Autodesk Inventor part; units mm, degrees
ref_plane "РабПлоскость1" through (-34.9448, 28.465, -130.3508) normal (0, 0, 1) x (1, 0, 0)
ref_plane "YZ Plane" through (0, 0, 0) normal (1, 0, 0) x (0, 1, 0)
ref_plane "XZ Plane" through (0, 0, 0) normal (0, 1, 0) x (-1, 0, 0)
ref_plane "РабПлоскость1" through (-34.9448, 28.465, -130.3508) normal (0, 0, 1) x (1, 0, 0)
sketch "Эскиз1" plane through (-34.9448, 28.465, -130.3508) normal (0, 0, 1) x (1, 0, 0)
  line L0 (0, 3.6904) -> (-12.8571, 3.6904) construction
  line L1 (0, 3.6904) -> (0, 9.6905)
  line L2 (-12.8571, 9.6905) -> (0, 9.6905)
  line L3 (-12.8571, 3.6904) -> (-12.8571, 9.6905)
  line L4 (25.7143, 3.6904) -> (12.8571, 3.6904) construction
  line L5 (25.7143, 3.6904) -> (25.7143, 9.6905)
  line L6 (12.8571, 9.6905) -> (25.7143, 9.6905)
  line L7 (12.8571, 3.6904) -> (12.8571, 9.6905)
  line L8 (51.4286, 3.6904) -> (38.5714, 3.6904) construction
  line L9 (51.4286, 3.6904) -> (51.4286, 9.6905)
  line L10 (38.5714, 9.6905) -> (51.4286, 9.6905)
  line L11 (38.5714, 3.6904) -> (38.5714, 9.6905)
  line L12 (77.1429, 3.6904) -> (64.2857, 3.6904) construction
  line L13 (77.1429, 3.6904) -> (77.1429, 9.6905)
  line L14 (64.2857, 9.6905) -> (77.1429, 9.6905)
  line L15 (64.2857, 3.6904) -> (64.2857, 9.6905)
  line L16 (0, 3.6904) -> (12.8571, 3.6904)
  line L17 (25.7143, 3.6904) -> (38.5714, 3.6904)
  line L18 (51.4286, 3.6904) -> (64.2857, 3.6904)
  line L19 (-12.8571, 3.6904) -> (-12.8571, -50.3096)
  line L20 (-9.8571, -53.3096) -> (-4.7353, -53.3096)
  line L21 (77.1429, 3.6904) -> (77.1429, -50.3096)
  line L22 (74.1429, -53.3096) -> (69.021, -53.3096)
  line L23 (-1.8571, -53.3096) -> (66.1429, -53.3096) construction
  arc A0 (-1.7452, -56.0663) -> (66.0309, -56.0663) centre (32.1429, -53.3096) ccw
  arc A1 (-1.7452, -56.0663) -> (-4.7353, -53.3096) centre (-4.7353, -56.3096) ccw
  arc A2 (69.021, -53.3096) -> (66.0309, -56.0663) centre (69.021, -56.3096) ccw
  arc A3 (74.1429, -53.3096) -> (77.1429, -50.3096) centre (74.1429, -50.3096) ccw
  arc A4 (-12.8571, -50.3096) -> (-9.8571, -53.3096) centre (-9.8571, -50.3096) ccw
  circle A5 centre (32.1429, -53.3095) radius 2.375
  point P0 (34.9448, -28.465)
  point P1 (77.1429, -53.3096)
  dimension "d0" = 57
  dimension "d1" = 34
  dimension "d2" = 3
  dimension "d3" = 6
  dimension "d14" = 4.75
ref_plane "РабПлоскость2" through (-162.802, 331.465, 111.3492) normal (0, 0, 1) x (1, 0, 0)
extrude "Выдавливание1" add sketch "Эскиз1" along normal blind 6
sketch "Эскиз6" plane through (-34.9448, 28.465, -130.3508) normal (0, 0, -1) x (-1, 0, 0)
  line L0 (-30.9731, -35.6894) -> (-30.9731, -26.6894)
  line L1 (-30.9731, -26.6894) -> (-26.9731, -26.6894)
  line L2 (-26.9731, -35.6894) -> (-30.9731, -35.6894)
  line L3 (-26.9731, -26.6894) -> (-26.9731, -35.6894)
  line L4 (-26.9731, 0.3106) -> (-26.9731, -8.6894)
  line L5 (-26.9731, -8.6894) -> (-30.9731, -8.6894)
  line L6 (-30.9731, 0.3106) -> (-26.9731, 0.3106)
  line L7 (-30.9731, -8.6894) -> (-30.9731, 0.3106)
extrude "Выдавливание5" cut sketch "Эскиз6" against normal blind 10
sketch "Эскиз2" plane through (-34.9448, 28.465, -130.3508) normal (0, 0, -1) x (-1, 0, 0)
  line L0 (-4.9286, 3.6904) -> (-4.9286, -2.6596)
  line L1 (-4.9286, -2.6596) -> (-3.6786, -2.6596)
  line L2 (-3.6786, -2.6596) -> (-3.6786, -4.9596)
  line L3 (-3.6786, -4.9596) -> (-4.9286, -4.9596)
  line L4 (-4.9286, -4.9596) -> (-4.9286, -11.3096)
  line L5 (-4.9286, -11.3096) -> (-7.9286, -11.3096)
  line L6 (-7.9286, -11.3096) -> (-7.9286, -4.9596)
  line L7 (-7.9286, -4.9596) -> (-9.1786, -4.9596)
  line L8 (-9.1786, -4.9596) -> (-9.1786, -2.6596)
  line L9 (-9.1786, -2.6596) -> (-7.9286, -2.6596)
  line L10 (-7.9286, -2.6596) -> (-7.9286, 3.6904)
  line L11 (-56.3571, 3.6904) -> (-59.3571, 3.6904)
  line L12 (-56.3571, 3.6904) -> (-56.3571, -2.6596)
  line L13 (-56.3571, -2.6596) -> (-55.1071, -2.6596)
  line L14 (-55.1071, -2.6596) -> (-55.1071, -4.9596)
  line L15 (-55.1071, -4.9596) -> (-56.3571, -4.9596)
  line L16 (-56.3571, -4.9596) -> (-56.3571, -11.3096)
  line L17 (-56.3571, -11.3096) -> (-59.3571, -11.3096)
  line L18 (-59.3571, -11.3096) -> (-59.3571, -4.9596)
  line L19 (-59.3571, -4.9596) -> (-60.6071, -4.9596)
  line L20 (-60.6071, -4.9596) -> (-60.6071, -2.6596)
  line L21 (-60.6071, -2.6596) -> (-59.3571, -2.6596)
  line L22 (-59.3571, -2.6596) -> (-59.3571, 3.6904)
  line L23 (-56.3571, 3.6904) -> (-59.3571, 3.6904)
  line L24 (-4.9286, 3.6904) -> (-7.9286, 3.6904)
  line L25 (-25.7143, 3.6904) -> (-25.7143, 9.6905)
  line L26 (-38.5714, 3.6904) -> (-25.7143, 3.6904)
  line L27 (-38.5714, 9.6905) -> (-38.5714, 3.6904)
  line L28 (-51.4286, 3.6904) -> (-51.4286, 9.6905)
  line L29 (-64.2857, 3.6904) -> (-51.4286, 3.6904)
  line L30 (-64.2857, 9.6905) -> (-64.2857, 3.6904)
  line L31 (-77.1429, -50.3096) -> (-77.1429, 9.6905)
  arc A0 (-77.1429, -50.3096) -> (-74.1429, -53.3096) centre (-74.1429, -50.3096) ccw
  line L32 (-69.021, -53.3096) -> (-74.1429, -53.3096)
  arc A1 (-66.0309, -56.0663) -> (-69.021, -53.3096) centre (-69.021, -56.3096) ccw
  arc A2 (-66.0309, -56.0663) -> (1.7452, -56.0663) centre (-32.1429, -53.3096) ccw
  arc A3 (4.7353, -53.3096) -> (1.7452, -56.0663) centre (4.7353, -56.3096) ccw
  line L33 (9.8571, -53.3096) -> (4.7353, -53.3096)
  arc A4 (9.8571, -53.3096) -> (12.8571, -50.3096) centre (9.8571, -50.3096) ccw
  line L34 (12.8571, 9.6905) -> (12.8571, -50.3096)
  line L35 (0, 3.6904) -> (0, 9.6905)
  line L36 (-12.8571, 3.6904) -> (0, 3.6904)
  line L37 (-12.8571, 9.6905) -> (-12.8571, 3.6904)
  circle A5 centre (-32.1429, -53.3095) radius 2.375
  line L38 (-25.7143, 9.6905) -> (-12.8571, 9.6905)
  line L39 (-51.4286, 9.6905) -> (-38.5714, 9.6905)
  line L40 (-77.1429, 9.6905) -> (-64.2857, 9.6905)
  line L41 (0, 9.6905) -> (12.8571, 9.6905)
  point P0 (-6.4286, 0)
sketch "Эскиз4" plane through (29.3409, 38.1554, -130.3508) normal (0, 1, 0) x (1, 0, 0)
  line L0 (-77.1429, 0) -> (-77.1429, -6)
  line L1 (12.8571, 0) -> (-77.1429, 0)
  line L2 (-77.1429, 0) -> (-77.1429, -6)
  line L3 (-77.1429, -6) -> (12.8571, -6)
  line L4 (12.8571, -6) -> (12.8571, 0)
  point P0 (-29.3409, -130.3508)
sketch "Эскиз5" plane through (-34.9448, 28.465, -130.3508) normal (0, 0, -1) x (-1, 0, 0)
  line L0 (-236.4804, 8.6905) -> (-77.1429, 8.6905) construction
  line L1 (-77.1429, 8.6905) -> (-64.2857, 8.6905) construction
  line L2 (-64.2857, 8.6905) -> (-51.4286, 8.6905) construction
  line L3 (-51.4286, 8.6905) -> (-38.5714, 8.6905) construction
  line L4 (-38.5714, 8.6905) -> (-25.7143, 8.6905) construction
  line L5 (-25.7143, 8.6905) -> (-12.8571, 8.6905) construction
  line L6 (-12.8571, 8.6905) -> (0, 8.6905) construction
  line L7 (0, 8.6905) -> (12.8571, 8.6905) construction
  line L8 (12.8571, 8.6905) -> (44.8254, 8.6905) construction
  line L9 (44.8254, 8.6905) -> (44.8254, 3.6905) construction
  line L10 (44.8254, 3.6905) -> (12.8571, 3.6905) construction
  line L11 (12.8571, 3.6905) -> (12.8571, 8.6905) construction
  line L12 (-236.4804, 3.6905) -> (-236.4804, 8.6905) construction
  line L13 (-77.1429, 3.6905) -> (-236.4804, 3.6905) construction
  line L14 (-64.2857, 3.6905) -> (-77.1429, 3.6905) construction
  line L15 (-51.4286, 3.6905) -> (-64.2857, 3.6905) construction
  line L16 (-38.5714, 3.6905) -> (-51.4286, 3.6905) construction
  line L17 (-25.7143, 3.6905) -> (-38.5714, 3.6905) construction
  line L18 (-12.8571, 3.6905) -> (-25.7143, 3.6905) construction
  line L19 (0, 3.6905) -> (-12.8571, 3.6905) construction
  line L20 (12.8571, 3.6905) -> (0, 3.6905) construction
  line L21 (-77.1429, 8.6905) -> (-77.1429, 3.6905) construction
  line L22 (-64.2857, 3.6905) -> (-64.2857, 8.6905) construction
  line L23 (-51.4286, 8.6905) -> (-51.4286, 3.6905) construction
  line L24 (-38.5714, 3.6905) -> (-38.5714, 8.6905) construction
  line L25 (-25.7143, 8.6905) -> (-25.7143, 3.6905) construction
  line L26 (-12.8571, 3.6905) -> (-12.8571, 8.6905) construction
  line L27 (0, 8.6905) -> (0, 3.6905) construction
  line L28 (-242.4804, 3.6905) -> (-352.8338, 3.6905) construction
  line L29 (-352.8338, 3.6905) -> (-352.8338, 8.6905) construction
  line L30 (-352.8338, 8.6905) -> (-242.4804, 8.6905) construction
  line L31 (-242.4804, 8.6905) -> (-242.4804, 3.6905) construction
  line L32 (-34.1429, 3.6915) -> (-30.1429, 3.6915) construction
  line L33 (-30.1429, -50.9345) -> (-34.1429, -50.9345) construction
  line L34 (-34.1429, 3.6915) -> (-30.1429, -50.9345) construction
  line L35 (-30.1429, 3.6915) -> (-34.1429, -50.9345) construction
  circle A0 centre (-32.1429, -53.3095) radius 2.375 construction
  line L36 (-34.1429, -5.6215) -> (-30.1429, -5.6215)
  line L37 (-30.1429, -41.6215) -> (-34.1429, -41.6215)
  line L38 (-34.1429, -5.6215) -> (-30.1429, -41.6215) construction
  line L39 (-30.1429, -5.6215) -> (-34.1429, -41.6215) construction
  line L40 (-34.1429, -14.6215) -> (-30.1429, -14.6215)
  line L41 (-30.1429, -32.6215) -> (-34.1429, -32.6215)
  line L42 (-34.1429, -14.6215) -> (-30.1429, -32.6215) construction
  line L43 (-30.1429, -14.6215) -> (-34.1429, -32.6215) construction
  line L44 (-34.1429, -41.6215) -> (-34.1429, -32.6215)
  line L45 (-34.1429, -14.6215) -> (-34.1429, -5.6215)
  line L46 (-30.1429, -5.6215) -> (-30.1429, -14.6215)
  line L47 (-30.1429, -32.6215) -> (-30.1429, -41.6215)
  line L48 (-30.1429, -32.6215) -> (-30.1429, -41.6215) construction
  line L49 (-34.1429, -50.9345) -> (-34.1429, -32.6215) construction
  line L50 (-34.1429, -14.6215) -> (-34.1429, 3.6915) construction
  line L51 (-30.1429, 3.6915) -> (-30.1429, 3.6905) construction
  line L52 (-30.1429, -5.6215) -> (-30.1429, -14.6215) construction
  point P0 (-34.9448, -28.465)
  point P1 (-32.1429, -23.6215)
  point P2 (-32.1429, -50.9345)
  dimension "d20" = 4
  dimension "d21" = 54.626
equation "\"d4\" = d3"
properties part number "wheel1"
Work out the finished part from the listing and answer in its coordinate system (mm). A direction names the side the tool comes from. Round coordinates to 2 decimals unless told otherwise and drop trailing zeros. Write each loop counter-clockwise with the first axis right and the second up, starting at its lowest first coordinate (ties: lowest second). Pieces come first, ordered by that corner, then holes.
1) A cutting plane is placed at D-D (y = -42). Give the vertices of the cut face in (x, z), plus the area to 3 significant figures.
2) A tool of negligible diameter and unlimited length cuts with its end or side. For faces 1 (the flat face through (-29, 32.155, -127)), 2 (the flat face through (37, -24.845, -127)), 3 (the flat face through (-42, -24.845, -127)), 4 (the flat face through (-3.972, -3, -127)), from which of +Z, -Z, +X, -X, +Y, -Y can it reach the whole face along a straight path? Write none if from no direction.
3) A cutting plane is placed at A-A (y = 26.5). Give the vertices of the cut face in (x, z), plus the area to 3 significant figures.
4) A cutting plane is placed at C-C (x = 19.5). Give the vertices of the cut face in (y, z), plus the area to 3 significant figures.
5) Straight lines are drawn through the part: line 1 (X direction, y = 22, z = -128.4); line 2 (Y direction, x = -44, z = -130.1); line 3 (X direction, y = -40, z = -129.55). For each, find the intervals that lie inside material, in ascending order.
6) Given pin 1 Ø3 at (x, z) = (20.5, -126) entering from +Y; pin 2 Ø2.5 at (x, z) = (37.5, -126.5) entering from -Y; pin 3 Ø1.5 at (y, z) = (-40, -126) entering from -X, each flat-ended and moving along its own axis, determine where each tip first touches the part or whether it passes through.
7) A cutting plane is placed at B-B (z = -129.3). Give the number of separate pieces and of enclosed holes in the cut face, plus the area to 3 significant figures.
8) The mould has two halves that part along Y. Classify faces 5 (the flat face through (-3, -10, -124.351)), 6 (the flat face through (-6, 1.776, -127)), 7 (the flat face through (36, 38.156, -127)), 8 (the flat face through (-3.972, 24, -127)): pulls with the +Y half, pulls with the -Y half, needs draft (parallel to the pull), parting line crosses it, or undercut.
Completed:
1. outline: (-32.16, -130.35) - (26.55, -130.35) - (26.55, -124.35) - (-32.16, -124.35) - close
1. area: 352 mm2
2. face 1: +Z, -Z, +Y
2. face 2: +Z, -Z, +X, -Y
2. face 3: +Z, -Z, -X, -Y
2. face 4: +Z, -Z
3. outline: (-47.8, -130.35) - (-7.97, -130.35) - (-7.97, -124.35) - (-47.8, -124.35) - close; (-3.97, -130.35) - (42.2, -130.35) - (42.2, -124.35) - (-3.97, -124.35) - close
3. area: 516 mm2
4. outline: (-50.51, -130.35) - (32.16, -130.35) - (32.16, -124.35) - (-50.51, -124.35) - close
4. area: 496 mm2
5. line 1: x = -47.8 to -7.97, -3.97 to 42.2
5. line 2: y = -24.84 to 38.16
5. line 3: x = -33.24 to 27.63
6. pin 1: stops at y = 32.16
6. pin 2: stops at y = -24.84
6. pin 3: stops at x = -33.6
7. separate pieces: 1
7. enclosed holes: 3
7. area: 7,160 mm2
8. face 5: needs draft
8. face 6: undercut
8. face 7: pulls with the +Y half
8. face 8: undercut
